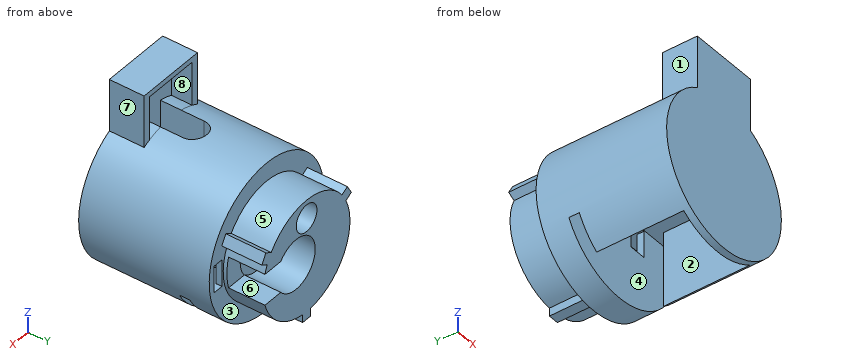
from build123d import *
from build123d.topology import SkipClean

# Parameters (mm, degrees)
SKETCH2_R                = 43
BOSS_EXTRUDE1_DEPTH      = 75
BOSS_EXTRUDE2_DEPTH      = 23
SKETCH4_R                = 14.5
CUT_EXTRUDE2_DEPTH       = 22.6
CUT_EXTRUDE3_START       = -20.9
CUT_EXTRUDE3_DEPTH       = 20.9
CUT_EXTRUDE6_START       = 4
CUT_EXTRUDE6_DEPTH       = 56
CUT_EXTRUDE6_START_2     = 54
CUT_EXTRUDE6_2_DEPTH     = 6
SKETCH8_W                = 6
SKETCH8_H                = 15.5
CUT_EXTRUDE7_DEPTH       = 13
SKETCH10_W               = 15.5
SKETCH10_H               = 7.5
CUT_EXTRUDE8_DEPTH       = 25
SKETCH12_W               = 10
SKETCH12_H               = 15.5
CUT_EXTRUDE9_DEPTH       = 8
SKETCH7_R                = 7.75
CUT_EXTRUDE10_DEPTH      = 90
BOSS_EXTRUDE3_DEPTH      = 20
CUT_EXTRUDE11_REACH      = 156.236
CUT_EXTRUDE12_REACH      = 156.236
CUT_EXTRUDE12_END_RADIUS = 43
SKETCH16_W               = 32
SKETCH16_H               = 12
SKETCH17_W               = 40
SKETCH17_H               = 20
BOSS_EXTRUDE4_DEPTH      = 3


# Read off the part's stored shape, not the designer's step: Cut-Extrude6
with BuildPart() as part:
    # Sketch2 → Boss-Extrude1 (new body)
    with BuildSketch(Plane(origin=(0, 0, 0), x_dir=(1, 0, 0), z_dir=(0, 1, 0))):
        with Locations(Location((0, 0, 0), (0, 0, 270))):
            Circle(SKETCH2_R)
    extrude(amount=BOSS_EXTRUDE1_DEPTH)

    # Sketch3 → Boss-Extrude2 (add)
    with BuildSketch(Plane(origin=(0, 75, 0), x_dir=(1, 0, 0), z_dir=(0, 1, 0))):
        with BuildLine():
            Line((-3, 32.361242251), (-3, 37))
            Line((-3, 37), (3, 37))
            Line((3, 37), (3, 32.361242251))
            ThreePointArc((3, 32.361242251), (28.145825623, 16.25), (29.525657887, -13.582544914))
            Line((29.525657887, -13.582544914), (33.54293994, -15.901923789))
            Line((33.54293994, -15.901923789), (30.54293994, -21.098076211))
            Line((30.54293994, -21.098076211), (26.525657887, -18.778697337))
            ThreePointArc((26.525657887, -18.778697337), (0, -32.5), (-26.525657887, -18.778697337))
            Line((-26.525657887, -18.778697337), (-30.54293994, -21.098076211))
            Line((-30.54293994, -21.098076211), (-33.54293994, -15.901923789))
            Line((-33.54293994, -15.901923789), (-29.525657887, -13.582544914))
            ThreePointArc((-29.525657887, -13.582544914), (-28.145825623, 16.25), (-3, 32.361242251))
        make_face()
    extrude(amount=BOSS_EXTRUDE2_DEPTH)

    # Sketch4 → Cut-Extrude2 (cut)
    with BuildSketch(Plane(origin=(0, 98, 0), x_dir=(1, 0, 0), z_dir=(0, 1, 0))):
        with Locations(Location((8, 0, 0), (0, 0, 270))):
            Circle(SKETCH4_R)
    extrude(amount=-CUT_EXTRUDE2_DEPTH, mode=Mode.SUBTRACT)

    # Sketch5 → Cut-Extrude3 (cut)
    with BuildSketch(Plane(origin=(0, 98, 0), x_dir=(1, 0, 0), z_dir=(0, 1, 0)).offset(CUT_EXTRUDE3_START)):
        with BuildLine():
            Line((19.368817001, 9), (31.228992939, 9))
            ThreePointArc((31.228992939, 9), (32.5, 0), (31.228992939, -9))
            Line((31.228992939, -9), (19.368817001, -9))
            ThreePointArc((19.368817001, -9), (22.5, 0), (19.368817001, 9))
        make_face()
    extrude(amount=CUT_EXTRUDE3_DEPTH, mode=Mode.SUBTRACT)

    # Cut-Extrude6 outline → Cut-Extrude6 (cut)
    with BuildSketch(Plane(origin=(0, 0, 0), x_dir=(1, 0, 0), z_dir=(0, 1, 0)).offset(CUT_EXTRUDE6_START)):
        with BuildLine():
            Line((-25, 34.985711369), (-25, -8))
            Line((-25, -8), (25, -8))
            Line((25, -8), (25, 34.985711369))
            ThreePointArc((25, 34.985711369), (0, 43), (-25, 34.985711369))
        make_face()
    extrude(amount=CUT_EXTRUDE6_DEPTH, mode=Mode.SUBTRACT)

    # Cut-Extrude6 2 outline → Cut-Extrude6 2 (cut)
    with BuildSketch(Plane(origin=(0, 0, 0), x_dir=(1, 0, 0), z_dir=(0, 1, 0)).offset(CUT_EXTRUDE6_START_2)):
        with BuildLine():
            Line((-38, 20.124611797), (-38, -8))
            Line((-38, -8), (-25, -8))
            Line((-25, -8), (-25, 34.985711369))
            ThreePointArc((-25, 34.985711369), (-32.36453414, 28.311427549), (-38, 20.124611797))
        make_face()
        with BuildLine():
            Line((25, 34.985711369), (25, -8))
            Line((25, -8), (38, -8))
            Line((38, -8), (38, 20.124611797))
            ThreePointArc((38, 20.124611797), (32.36453414, 28.311427549), (25, 34.985711369))
        make_face()
    extrude(amount=CUT_EXTRUDE6_2_DEPTH, mode=Mode.SUBTRACT)

    # Sketch8 → Cut-Extrude7 (cut)
    with BuildSketch(Plane(origin=(0, 77.1, 0), x_dir=(1, 0, 0), z_dir=(0, 1, 0))):
        with Locations((36.5, 0)):
            Rectangle(SKETCH8_W, SKETCH8_H)
    extrude(amount=-CUT_EXTRUDE7_DEPTH, mode=Mode.SUBTRACT)

    # Sketch10 → Cut-Extrude8 (cut)
    with BuildSketch(Plane(origin=(33.5, 0, 0), x_dir=(0, 0, -1), z_dir=(1, 0, 0))):
        with Locations((0, 67.85)):
            Rectangle(SKETCH10_W, SKETCH10_H)
    extrude(amount=-CUT_EXTRUDE8_DEPTH, mode=Mode.SUBTRACT)

    # Sketch12 → Cut-Extrude9 (cut)
    with BuildSketch(Plane(origin=(0, 64.1, 0), x_dir=(1, 0, 0), z_dir=(0, 1, 0))):
        with Locations((13.5, 0)):
            Rectangle(SKETCH12_W, SKETCH12_H)
    extrude(amount=-CUT_EXTRUDE9_DEPTH, mode=Mode.SUBTRACT)

    # Sketch7 → Cut-Extrude10 (cut)
    with BuildSketch(Plane(origin=(0, 98, 0), x_dir=(1, 0, 0), z_dir=(0, 1, 0))):
        with Locations(Location((0, -22, 0), (0, 0, 270))):
            Circle(SKETCH7_R)
    extrude(amount=-CUT_EXTRUDE10_DEPTH, mode=Mode.SUBTRACT)

    # Sketch13 → Boss-Extrude3 (add)
    with BuildSketch(Plane.XZ):
        with BuildLine():
            Line((-20, 38.065732621), (-20, 68.065732621))
            Line((-20, 68.065732621), (20, 68.065732621))
            Line((20, 68.065732621), (20, 38.065732621))
            ThreePointArc((20, 38.065732621), (0, 43), (-20, 38.065732621))
        make_face()
    extrude(amount=-BOSS_EXTRUDE3_DEPTH)

    # Sketch14 → Cut-Extrude11 (cut, up to next)
    with BuildSketch(Plane.XY.offset(68.065732621), mode=Mode.PRIVATE) as cut_extrude11_sk1:
        with BuildLine():
            Line((-7.75, 8), (7.75, 8))
            Line((7.75, 8), (7.75, 33.050905548))
            ThreePointArc((7.75, 33.050905548), (0, 40.750167184), (-7.75, 33.050905548))
            Line((-7.75, 33.050905548), (-7.75, 8))
        make_face()
    cut_extrude11_tool1 = extrude(cut_extrude11_sk1.sketch, amount=-CUT_EXTRUDE11_REACH, mode=Mode.PRIVATE) & part.part
    add(cut_extrude11_tool1.solids().sort_by_distance((0, 23.591664, 68.065733))[0], mode=Mode.SUBTRACT)

    # Cut-Extrude12: up to this cylinder (the profile starts outside it)
    with SkipClean():  # the faces are left unmerged after this step: merging them gives an invalid solid
        cut_extrude12_end = Plane(origin=(0, 14, 0), z_dir=(0, -1, 0)) * Cylinder(CUT_EXTRUDE12_END_RADIUS, 399.472, mode=Mode.PRIVATE)
        # Sketch16 → Cut-Extrude12 (cut, up to the surface)
        with BuildSketch(Plane.XY.offset(68.065732621), mode=Mode.PRIVATE) as cut_extrude12_sk1:
            with Locations((0, 14)):
                Rectangle(SKETCH16_W, SKETCH16_H)
        cut_extrude12_tool1 = extrude(cut_extrude12_sk1.sketch, amount=-CUT_EXTRUDE12_REACH, mode=Mode.PRIVATE) - cut_extrude12_end
        add(cut_extrude12_tool1.solids().sort_by_distance((0, 14, 68.065733))[0], mode=Mode.SUBTRACT)

    # Sketch17 → Boss-Extrude4 (add)
    with SkipClean():  # the faces are left unmerged after this step: merging them gives an invalid solid
        with BuildSketch(Plane.XY.offset(68.065732621)):
            with Locations((0, 10)):
                Rectangle(SKETCH17_W, SKETCH17_H)
        extrude(amount=-BOSS_EXTRUDE4_DEPTH)


solid = part.part
Geometry: final body of the model. Coordinates: model frame, mm. Face numbers are marked on the shaded views. A direction names the side the tool comes from. Round coordinates to 2 decimals unless told otherwise and drop trailing zeros. Loops run counter-clockwise (first coordinate to the right, second up) from the corner with the lowest first, then second, coordinate; pieces in that order, holes last.
Q1. Section A-A on z = 0. Return loops of the section in (x, y), plus the area to 3 significant figures.
Q2. Section C-C on z = -25. Return loops of the section in (x, y), plus the area to 3 significant figures.
Q3. Material intervals for L1, parallel to Y at x = -3.5, z = -27; L2, parallel to Y at x = 21.5, z = 6; L3, parallel to Z at x = 3.5, y = 78, sorted ascending.
Q4. Pull-direction query (Y, two-part tool) for the marked faces 1, 2, 3 and 4; classes: released by +Y, released by -Y, zero draft, split by the parting line, or undercut.
Q5. Pin query (flat end, axial travel): P1, Ø8, axis at x = -6.5, y = 16, coming from the -Z side; P2, Ø4.5, axis at x = 31, y = 65.5, coming from the +Z side; P3, Ø1.8, axis at y = 56, z = -0.5, coming from the +X side. Return the tip coordinate at first contact, or that it passes through.
Q6. Access query for the marked faces 5, 6, 7 and 8. Directions: +Z, -Z, +X, -X, +Y, -Y. A direction counts if a zero-diameter tool reaches every point of the face in a straight line with its end or side. Return the directions, or none.
Q7. Section D-D on x = 0. Return loops of the section in (y, z), plus the area to 3 significant figures.
Q8. Section B-B on y = 86.5. Return loops of the section in (x, z).
Evaluation:
1. outline: (-43, 0) - (43, 0) - (43, 75) - (39.5, 75) - (39.5, 64.1) - (18.5, 64.1) - (18.5, 60) - (38, 60) - (38, 54) - (25, 54) - (25, 4) - (-25, 4) - (-25, 54) - (-38, 54) - (-38, 60) - (8.5, 60) - (8.5, 71.6) - (33.5, 71.6) - (33.5, 75) - (32.5, 75) - (32.5, 77.1) - (22.5, 77.1) - (22.5, 75.4) - (-6.5, 75.4) - (-6.5, 98) - (-32.5, 98) - (-32.5, 75) - (-43, 75) - close
1. area: 3,830 mm2
2. outline: (-34.99, 0) - (34.99, 0) - (34.99, 54) - (25, 54) - (25, 4) - (-25, 4) - (-25, 54) - (-34.99, 54) - close; (-34.99, 60) - (34.99, 60) - (34.99, 75) - (20.77, 75) - (20.77, 98) - (-20.77, 98) - (-20.77, 75) - (-34.99, 75) - close
2. area: 3,280 mm2
3. L1: y = 0 to 4, 60 to 98
3. L2: y = 0 to 4, 60 to 64.1, 71.6 to 77.1
3. L3: z = -32.31 to -13.78, 13.78 to 15.09, 28.91 to 32.31
4. face 1: zero draft
4. face 2: undercut
4. face 3: released by +Y
4. face 4: undercut
5. P1: stops at z = 8
5. P2: stops at z = 31.98
5. P3: stops at x = 43
6. face 5: +Z, +Y
6. face 6: +X, +Y
6. face 7: +Z, +X, +Y, -Y
6. face 8: +Y
7. outline: (0, -43) - (4, -43) - (4, 8) - (60, 8) - (60, -43) - (75, -43) - (75, -37) - (98, -37) - (98, -12.09) - (75.4, -12.09) - (75.4, 12.09) - (98, 12.09) - (98, 14.25) - (8, 14.25) - (8, 65.07) - (20, 65.07) - (20, 68.07) - (0, 68.07) - close; (40.75, 29.75) - (98, 29.75) - (98, 32.5) - (75, 32.5) - (75, 43) - (40.75, 43) - close
7. area: 3,050 mm2
8. outline: (-33.54, 15.9) - (-29.53, 13.58) arc R32.5 ccw to (-3, -32.36) - (-3, -37) - (3, -37) - (3, -32.36) arc R32.5 ccw to (31.23, -9) - (19.37, -9) arc R14.5 cw (long way) to (19.37, 9) - (31.23, 9) arc R32.5 ccw to (29.53, 13.58) - (33.54, 15.9) - (30.54, 21.1) - (26.53, 18.78) arc R32.5 ccw to (-26.53, 18.78) - (-30.54, 21.1) - close; hole circle Ø15.5 at (0, 22)
